```python
from build123d import *

# Parameters (mm, degrees)
F4_R          = 4.5
F4_R_2        = 2
F5_DEPTH      = 9
F6_W          = 70.3
F6_H          = 35.0108387947
F6_W_2        = 50.3
F6_H_2        = 15.0108387947
F7_DEPTH      = 6
F8_R          = 4.5
F8_R_2        = 2
F9_DEPTH      = 5
F10_R         = 2
F11_DEPTH     = 9.001
F13_START     = -5
F12_R         = 3.5
F12_R_2       = 2
F13_DEPTH     = 23
F14_R         = 2
F15_DEPTH     = 9.001
F16_T1_DEPTH  = 6
F16_T3_DEPTH  = 6
F16_T5_DEPTH  = 6
F16_T7_DEPTH  = 6
F16_T9_DEPTH  = 31
F16_T14_DEPTH = 21.2263176167
F16_T19_DEPTH = 21.2263176167
F16_S20_R     = 4.5
F16_T21_DEPTH = 12
F16_T22_DEPTH = 31


# Not quite as in the source:
# - a fillet or chamfer that OpenCascade refuses, or shapes differently, is made with other operations: its cross-section is extruded or revolved along the edge and cut away or added
# - after a boolean that leaves OpenCascade's solid faulty, fix() repairs it


with BuildPart() as f5:
    # F4 (on Top) → F5 (new body)
    with BuildSketch(Plane.XY):
        with Locations((-30.4, 10.8)):
            Circle(F4_R)
        with Locations((-30.4, 10.8)):
            Circle(F4_R_2, mode=Mode.SUBTRACT)
    extrude(amount=F5_DEPTH)



with BuildPart() as f5b:
    # F4 (on Top) → F5, piece 2 (new body)
    with BuildSketch(Plane.XY):
        with Locations((30.9, -10.8)):
            Circle(F4_R)
        with Locations((30.9, -10.8)):
            Circle(F4_R_2, mode=Mode.SUBTRACT)
    extrude(amount=F5_DEPTH)


with BuildPart() as f5_1:
    add(f5.part)

    add(f5b.part)  # F7 merges F5b
    # F6 (on face) → F7 (join)
    with BuildSketch(Plane.XY):
        with Locations((0.25, 2.2054193974)):
            Rectangle(F6_W, F6_H)
        with Locations((0.25, 2.2054193974)):
            Rectangle(F6_W_2, F6_H_2, mode=Mode.SUBTRACT)
    extrude(amount=F7_DEPTH)

    # F8 (on face) → F9 (join)
    with BuildSketch(Plane.XY.offset(9)):
        with BuildLine():
            Line((-19.1311288741, -12.8), (-15.1, -12.8))
            Line((-15.1, -12.8), (-11.0688711259, -12.8))
            ThreePointArc((-11.0688711259, -12.8), (-10.7187855603, -11.8271124735), (-10.6, -10.8))
            ThreePointArc((-10.6, -10.8), (-16.1271124735, -6.4187855603), (-19.1311288741, -12.8))
        make_face()
        with BuildLine():
            ThreePointArc((-15.1, -12.8), (-16.5142135624, -9.3857864376), (-13.1, -10.8))
            ThreePointArc((-13.1, -10.8), (-13.6857864376, -12.2142135624), (-15.1, -12.8))
        make_face(mode=Mode.SUBTRACT)
        with BuildLine():
            Line((-11.0688711259, -12.8), (-15.1, -12.8))
            Line((-15.1, -12.8), (-19.1311288741, -12.8))
            ThreePointArc((-19.1311288741, -12.8), (-15.1, -15.3), (-11.0688711259, -12.8))
        make_face()
        with Locations((-15.1, 20.2)):
            Circle(F8_R)
        with Locations((-15.1, 20.2)):
            Circle(F8_R_2, mode=Mode.SUBTRACT)
        with Locations((30.9, 20.2)):
            Circle(F8_R)
        with Locations((30.9, 20.2)):
            Circle(F8_R_2, mode=Mode.SUBTRACT)
    extrude(amount=-F9_DEPTH)

    # F10 (on face) → F11 (cut, through all)
    with BuildSketch(Plane.XY.offset(9)):
        with Locations((30.9, -10.8)):
            Circle(F10_R)
        with Locations((-30.4, 10.8)):
            Circle(F10_R)
    extrude(amount=-F11_DEPTH, mode=Mode.SUBTRACT)

    # F12 (on face) → F13 (cut)
    with BuildSketch(Plane.XY.offset(9).offset(F13_START)):
        with Locations((-15.1, 20.2)):
            Circle(F12_R)
        with Locations((-15.1, 20.2)):
            Circle(F12_R_2, mode=Mode.SUBTRACT)
        with Locations((30.9, 20.2)):
            Circle(F12_R)
        with Locations((30.9, 20.2)):
            Circle(F12_R_2, mode=Mode.SUBTRACT)
        with Locations((-15.1, -10.8)):
            Circle(F12_R)
        with Locations((-15.1, -10.8)):
            Circle(F12_R_2, mode=Mode.SUBTRACT)
    extrude(amount=-F13_DEPTH, mode=Mode.SUBTRACT)

    # F14 (on face) → F15 (cut, through all)
    with BuildSketch(Plane.XY.offset(9)):
        with Locations((-15.1, 20.2)):
            Circle(F14_R)
        with Locations((30.9, 20.2)):
            Circle(F14_R)
        with Locations((-15.1, -10.8)):
            Circle(F14_R)
        with Locations((30.9, -10.8)):
            Circle(F14_R)
    extrude(amount=-F15_DEPTH, mode=Mode.SUBTRACT)

    add(f5_1.part.fix(), mode=Mode.REPLACE)

    # F16: fillet of radius 5 on 7 edges, made by hand

    # F16_s2 → F16_t1 (join)
    with BuildSketch(Plane.XY):
        with BuildLine():
            ThreePointArc((-24.9, -0.3), (-23.4355339059, -3.8355339059), (-19.9, -5.3))
            Line((-19.9, -5.3), (-24.9, -5.3))
            Line((-24.9, -5.3), (-24.9, -0.3))
        make_face()
    extrude(amount=F16_T1_DEPTH)

    # F16_s4 → F16_t3 (join)
    with BuildSketch(Plane.XY):
        with BuildLine():
            ThreePointArc((-24.9, 4.7108387947), (-23.4355339059, 8.2463727006), (-19.9, 9.7108387947))
            Line((-19.9, 9.7108387947), (-24.9, 9.7108387947))
            Line((-24.9, 9.7108387947), (-24.9, 4.7108387947))
        make_face()
    extrude(amount=F16_T3_DEPTH)

    # F16_s6 → F16_t5 (join)
    with BuildSketch(Plane.XY):
        with BuildLine():
            ThreePointArc((25.4, -0.3), (23.9355339059, -3.8355339059), (20.4, -5.3))
            Line((20.4, -5.3), (25.4, -5.3))
            Line((25.4, -5.3), (25.4, -0.3))
        make_face()
    extrude(amount=F16_T5_DEPTH)

    # F16_s8 → F16_t7 (join)
    with BuildSketch(Plane.XY):
        with BuildLine():
            ThreePointArc((25.4, 4.7108387947), (23.9355339059, 8.2463727006), (20.4, 9.7108387947))
            Line((20.4, 9.7108387947), (25.4, 9.7108387947))
            Line((25.4, 9.7108387947), (25.4, 4.7108387947))
        make_face()
    extrude(amount=F16_T7_DEPTH)

    # F16_s10 → F16_t9 (cut)
    with BuildSketch(Plane.XY.offset(-12.5)):
        with BuildLine():
            ThreePointArc((-34.9, -10.3), (-33.4355339059, -13.8355339059), (-29.9, -15.3))
            Line((-29.9, -15.3), (-34.9, -15.3))
            Line((-34.9, -15.3), (-34.9, -10.3))
        make_face()
    extrude(amount=F16_T9_DEPTH, mode=Mode.SUBTRACT)


with BuildPart() as f16_tool12:
    # F16_s13 → F16_t14 (new body)
    with BuildSketch(Plane.XY.offset(-7.6131588083)):
        with BuildLine():
            ThreePointArc((34.3656487582, 19.7108387947), (35.1343554889, 18.2736418448), (35.4, 16.6655752714))
            Line((35.4, 16.6655752714), (35.4, 19.7108387947))
            Line((35.4, 19.7108387947), (34.3656487582, 19.7108387947))
        make_face()
    extrude(amount=F16_T14_DEPTH)

    split(bisect_by=Plane.XY.offset(4), keep=Keep.BOTTOM)


with BuildPart() as f5_2:
    add(f5_1.part)

    # F16_t11: cut F16_tool12
    add(f16_tool12.part, mode=Mode.SUBTRACT)


with BuildPart() as f16_tool17:
    # F16_s18 → F16_t19 (new body)
    with BuildSketch(Plane.XY.offset(-7.6131588083)):
        with BuildLine():
            ThreePointArc((34.3656487582, 19.7108387947), (35.1343554889, 18.2736418448), (35.4, 16.6655752714))
            Line((35.4, 16.6655752714), (35.4, 19.7108387947))
            Line((35.4, 19.7108387947), (34.3656487582, 19.7108387947))
        make_face()
    extrude(amount=F16_T19_DEPTH)

    # F16_s20 → F16_t21 (cut, symmetric)
    with BuildSketch(Plane.XY.offset(3)):
        with Locations((30.9, 20.2)):
            Circle(F16_S20_R)
    extrude(amount=F16_T21_DEPTH, both=True, mode=Mode.SUBTRACT)


with BuildPart() as f5_3:
    add(f5_2.part)

    # F16_t16: cut F16_tool17
    add(f16_tool17.part, mode=Mode.SUBTRACT)

    # F16_s23 → F16_t22 (cut)
    with BuildSketch(Plane.XY.offset(-12.5)):
        with BuildLine():
            ThreePointArc((-29.9, 19.7108387947), (-33.4355339059, 18.2463727006), (-34.9, 14.7108387947))
            Line((-34.9, 14.7108387947), (-34.9, 19.7108387947))
            Line((-34.9, 19.7108387947), (-29.9, 19.7108387947))
        make_face()
    extrude(amount=F16_T22_DEPTH, mode=Mode.SUBTRACT)


solid = f5_3.part
```
Model file for the job. Use its own axes, mm. A direction names the side the tool comes from. Round coordinates to 2 decimals unless told otherwise and drop trailing zeros. Write each loop counter-clockwise with the first axis right and the second up, starting at its lowest first coordinate (ties: lowest second). Pieces come first, ordered by that corner, then holes. Notation, with made-up numbers: (88, 49.5) - (102, 49.5) arc R23 cw to (102, 57.5) - close; hole circle Ø4 at (31.5, 36). An arc over 180 degrees is marked (long way). One line per item, written item: value.
(1) Cut at B-B, the plane z = 7.25. Give the number of separate pieces and of enclosed holes in the cut face, plus the area to 3 significant figures.
Values follow:
separate pieces: 5
enclosed holes: 5
area: 255 mm²
(2) Cut at A-A, the plane x = 18.5. Give the cut face in (y, z).
Values follow:
outline: (-15.3, 0) - (-5.3, 0) - (-5.3, 6) - (-15.3, 6) - close; (9.71, 0) - (19.71, 0) - (19.71, 6) - (9.71, 6) - close
(3) Drop flat-ended pins along their axis: P1, Ø9, axis at x = -14.5, y = 20, coming from the -Z side; P2, Ø5, axis at x = -23.5, z = 3, coming from the +Y side; P3, Ø4.5, axis at x = 30.9, y = 20.2, coming from the -Z side; P4, Ø4, axis at x = 23, y = -6.5, coming from the +Z side. Give the stop position or say it passes through.
Values follow:
P1: stops at z = 0
P2: stops at y = 19.71
P3: stops at z = 4
P4: stops at z = 6
(4) Cut at D-D, the plane z = 2.5. Give the cut face in (x, y).
Values follow:
outline: (-34.9, -10.3) arc R5 ccw to (-29.9, -15.3) - (35.4, -15.3) - (35.4, 16.67) arc R5 ccw to (34.37, 19.71) arc R3.5 cw to (27.43, 19.71) - (-11.63, 19.71) arc R3.5 cw to (-18.57, 19.71) - (-29.9, 19.71) arc R5 ccw to (-34.9, 14.71) - close; hole circle Ø4 at (-30.4, 10.8); hole (-24.9, -0.3) arc R5 ccw to (-19.9, -5.3) - (20.4, -5.3) arc R5 ccw to (25.4, -0.3) - (25.4, 4.71) arc R5 ccw to (20.4, 9.71) - (-19.9, 9.71) arc R5 ccw to (-24.9, 4.71) - close; hole circle Ø7 at (-15.1, -10.8); hole circle Ø4 at (30.9, -10.8)
(5) Cut at C-C, the plane y = 4. Give the cut face in (x, z).
Values follow:
outline: (-34.9, 0) - (-24.9, 0) - (-24.9, 6) - (-34.9, 6) - close; (25.4, 0) - (35.4, 0) - (35.4, 6) - (25.4, 6) - close
(6) Wall check: probe 1 along Y at (x, z) = (-15.1, 8.25); probe 2 along Y at (x, z) = (-15.1, 4.5); probe 3 along Y at (x, z) = (-30.4, 6.25). Give the ranges that are in metal, low to high.
Values follow:
probe 1: y = -15.3 to -12.8, -8.8 to -6.3, 15.7 to 18.2, 22.2 to 24.7
probe 2: y = -15.3 to -12.8, -8.8 to -5.3, 9.71 to 18.2, 22.2 to 24.7
probe 3: y = 6.3 to 8.8, 12.8 to 15.3
(7) Two-plate mould, pull along Y, no slides. Class faces 6 (the flat face through (-34.9, 2, 3)), 7 (the cylindrical face through (-13.253, 19.434, 6.535)), 8 (the cylindrical face through (-33.396, 18.285, 2.958)): pulls with the +Y half, pulls with the -Y half, needs draft (parallel to the pull), parting line crosses it, or undercut.
Values follow:
face 6: needs draft
face 7: undercut
face 8: pulls with the +Y half
(8) 3-axis set-ups, long thin cutter, end or side, ignore diameter. For faces 1 (the flat face through (31, 23, 4)), 2 (the flat face through (34.5, -14.4, 6)), 3 (the cylindrical face through (-33.72, 13.84, 7.48)), 4 (the flat face through (25.4, 2, 3)), 5 (the flat face through (-15, -13, 4)): which of +Z, -Z, +X, -X, +Y, -Y reach the whole face in a straight line?
Values follow:
face 1: -Z, +Y
face 2: +Z, +X, -Y
face 3: +Z
face 4: +Z, -Z
face 5: -Z
